Could you check a few things on this drawing? It's one solid part, dimensions in mm from its lowest x, y, z. Give positions to 0.01 mm unless a question says otherwise; leave off trailing zeros. Write each loop counter-clockwise with the first axis right and the second up, starting at its lowest first coordinate (ties: lowest second). Pieces come first, ordered by that corner, then holes.
1. If I drill on probe 1 along Z at (x, y) = (41.25, 5) (3 decimals); probe 2 along X at (y, z) = (8, 63.5) (3 decimals); probe 3 along Z at (x, y) = (85.5, 6.5), over which ranges is the centre line in solid material (lowest first)?
2. Suppose I cut it at D-D (x = 41.25). Please give me the cut outline in (y, z) (3 decimals).
3. Suppose I cut it at C-C (y = 9). Please give me the cut outline in (x, z) (3 decimals).
4. I'm going to push a flat-ended pin straight in: pin 1 (2.5 mm diameter, centred on y = 6.5, z = 198, fed in from -X). Where does the tip first touch, or does it pass through?
5. Suppose I cut it at A-A (x = 87.5). Please give me the cut outline in (y, z).
6. Suppose I cut it at B-B (z = 63.5). Please give me the cut outline in (x, y) (3 decimals), and give its area (3 significant figures).
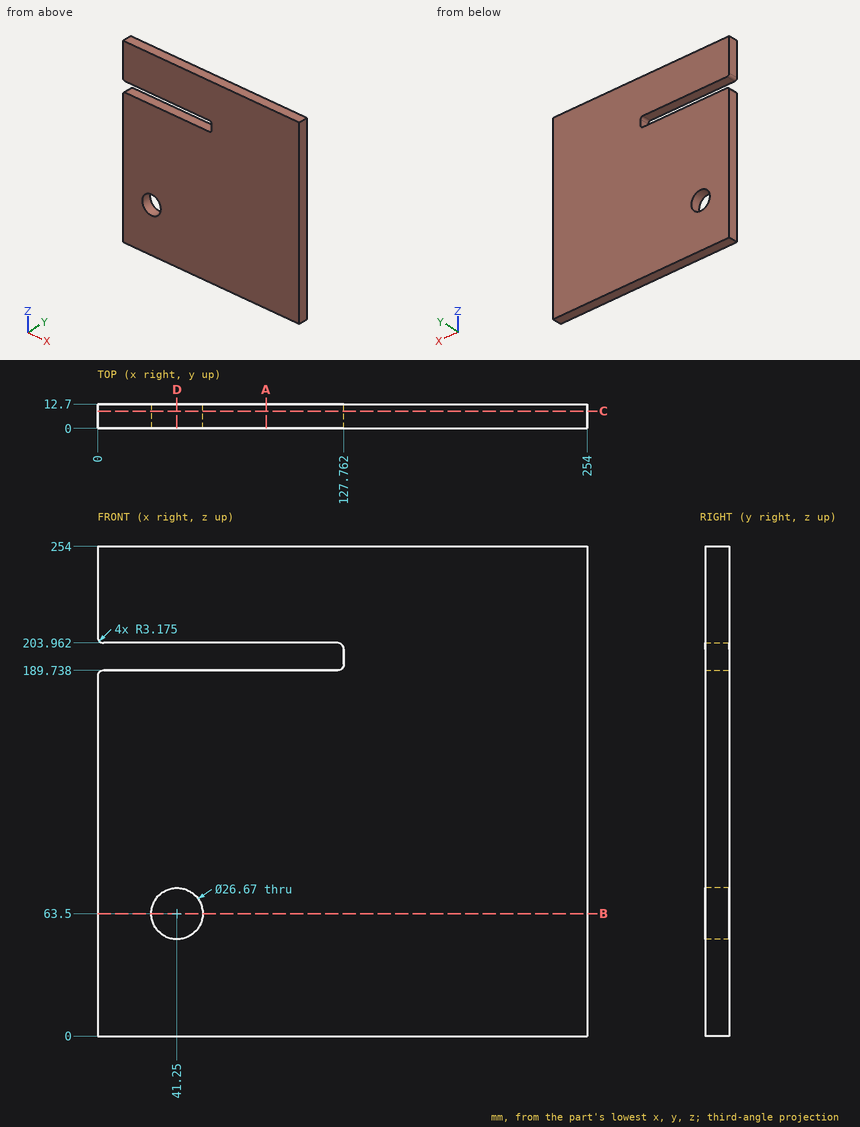
Checks:
1. probe 1: z = 0 to 50.165, 76.835 to 189.738, 203.962 to 254
1. probe 2: x = 0 to 27.915, 54.585 to 254
1. probe 3: z = 0 to 189.74, 203.96 to 254
2. outline: (0, 0) - (12.7, 0) - (12.7, 50.165) - (0, 50.165) - close; (0, 76.835) - (12.7, 76.835) - (12.7, 189.738) - (0, 189.738) - close; (0, 203.962) - (12.7, 203.962) - (12.7, 254) - (0, 254) - close
3. outline: (0, 0) - (254, 0) - (254, 254) - (0, 254) - (0, 207.137) arc R3.175 ccw to (3.175, 203.962) - (124.587, 203.962) arc R3.175 cw to (127.762, 200.787) - (127.762, 192.913) arc R3.175 cw to (124.587, 189.738) - (3.175, 189.738) arc R3.175 ccw to (0, 186.563) - close; hole circle Ø26.67 at (41.25, 63.5)
4. pin 1: stops at x = 127.76
5. outline: (0, 0) - (12.7, 0) - (12.7, 189.74) - (0, 189.74) - close; (0, 203.96) - (12.7, 203.96) - (12.7, 254) - (0, 254) - close
6. outline: (0, 0) - (27.915, 0) - (27.915, 12.7) - (0, 12.7) - close; (54.585, 0) - (254, 0) - (254, 12.7) - (54.585, 12.7) - close
6. area: 2,890 mm2
